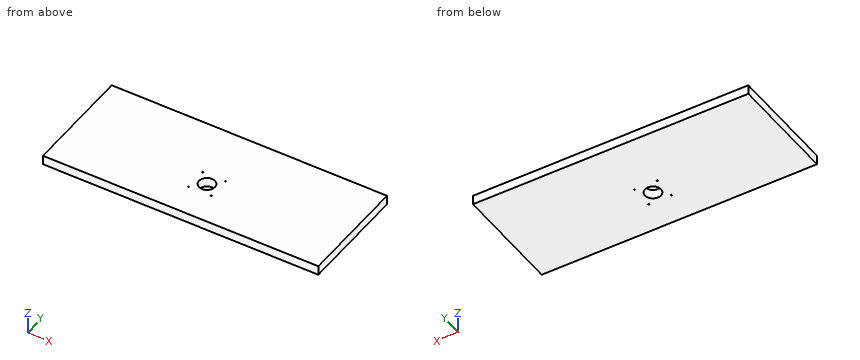
Autodesk Inventor part; units mm, degrees
ref_plane "YZ Plane" through (0, 0, 0) normal (1, 0, 0) x (0, 1, 0)
ref_plane "XZ Plane" through (0, 0, 0) normal (0, 1, 0) x (-1, 0, 0)
ref_plane "XY Plane" through (0, 0, 0) normal (0, 0, 1) x (1, 0, 0)
sketch "Sketch1" plane through (0, 0, 0) normal (0, 0, 1) x (1, 0, 0)
  line L0 (-191, 76.2) -> (191, 76.2)
  line L1 (191, 76.2) -> (191, -76.2)
  line L2 (191, -76.2) -> (-191, -76.2)
  line L3 (-191, -76.2) -> (-191, 76.2)
  line L4 (-191, 76.2) -> (191, -76.2) construction
  line L5 (191, 76.2) -> (-191, -76.2) construction
  point P0 (0, 0)
  dimension "d0" = 152.4
  dimension "d1" = 382
extrude "Extrusion1" add sketch "Sketch1" along normal mid plane 13
sketch "Sketch3" plane through (0, 0, 6.5) normal (0, 0, 1) x (1, 0, 0)
  circle A0 centre (15.76, -1.94) radius 0.8126
  circle A1 centre (-15.76, -1.94) radius 0.8126
  circle A2 centre (15.76, -33.46) radius 0.8126
  circle A3 centre (-15.76, -33.46) radius 0.8126
  line L0 (-15.76, -1.94) -> (15.76, -1.94)
  line L1 (15.76, -1.94) -> (15.76, -33.46)
  line L2 (15.76, -33.46) -> (-15.76, -33.46)
  line L3 (-15.76, -33.46) -> (-15.76, -1.94)
  line L4 (-15.76, -1.94) -> (15.76, -33.46) construction
  line L5 (15.76, -1.94) -> (-15.76, -33.46) construction
  line L6 (-191, -76.2) -> (191, -76.2)
  line L7 (-191, 76.2) -> (-191, -76.2)
  point P0 (0, 0)
  point P1 (0, -17.7)
  point P2 (0, -17.7)
  dimension "d5" = 31.52
  dimension "d6" = 31.52
  dimension "d7" = 58.5
hole "Hole1" at (15.76, -1.94, 6.5) at (-15.76, -1.94, 6.5) at (-15.76, -33.46, 6.5) at (15.76, -33.46, 6.5) direction (0, 0, -1) diameter 1.6252 end through all
sketch "Sketch4" plane through (0, 0, 6.5) normal (0, 0, 1) x (1, 0, 0)
  circle A0 centre (-15.76, -1.94) radius 0.8126
  circle A1 centre (15.76, -33.46) radius 0.8126
  circle A2 centre (0, -17.7) radius 11
  point P0 (0, 0)
  dimension "d18" = 22
hole "Hole2" at (0, -17.7, 6.5) direction (0, 0, -1) diameter 22 end through all
properties part number "CNC-X-axis- foundation faces"
Work out the finished part from the listing and answer in its coordinate system (mm). Give positions to 0.01 mm unless a question says otherwise; leave off trailing zeros. Loops run counter-clockwise (first coordinate to the right, second up) from the corner with the lowest first, then second, coordinate; pieces in that order, holes last. Notation, with made-up numbers: (1.5, 45.5) -> (53.5, 45.5) arc R25 ccw to (53.5, 66.5) -> close; hole circle Ø10 at (-22.5, -17.75). An arc over 180 degrees is marked (long way). Put each result on its own line as item: value. Start each with the question number.
Item 1: Find the intervals of material crossed by L1, parallel to X at y = -33.46, z = -3.5; L2, parallel to Y at x = -15.76, z = 1.25; L3, parallel to Y at x = 0, z = -3.5, in increasing order. Write a range as [from, to].
Item 2: The part is cut by section A-A (x = 0). Give the vertices of the cut face in (y, z), then the cut area to 3 significant figures.
Item 3: This flat-tipped pin is pushed along its axis until it touches: P1, Ø13, axis at x = 0, y = -17.7, coming from the -Z side. Where does it stop, or does it pass through?
Answers below:
1. L1: [-191, -16.57], [-14.95, 14.95], [16.57, 191]
1. L2: [-76.2, -34.27], [-32.65, -2.75], [-1.13, 76.2]
1. L3: [-76.2, -28.7], [-6.7, 76.2]
2. outline: (-76.2, -6.5) -> (-28.7, -6.5) -> (-28.7, 6.5) -> (-76.2, 6.5) -> close; (-6.7, -6.5) -> (76.2, -6.5) -> (76.2, 6.5) -> (-6.7, 6.5) -> close
2. area: 1,700 mm2
3. P1: through
